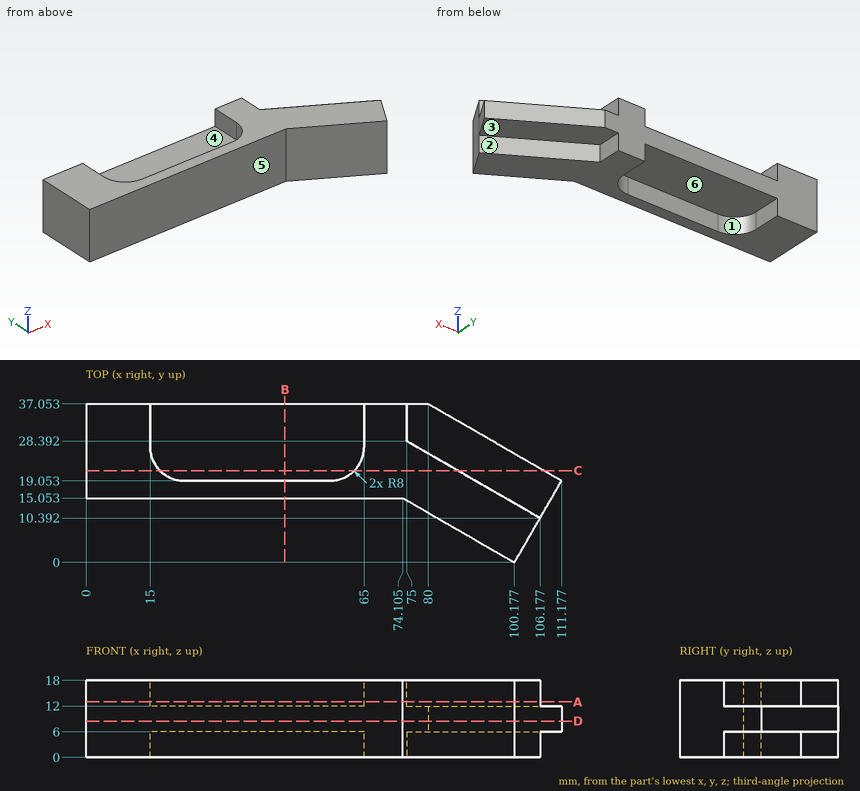
Can you work these out from the drawing? Everything is in mm from the part's minimum corner. A direction names the side the tool comes from. Round coordinates to 2 decimals unless told otherwise and drop trailing zeros. Loops run counter-clockwise (first coordinate to the right, second up) from the corner with the lowest first, then second, coordinate; pieces in that order, holes last. Notation, with made-up numbers: (-40, 68.25) - (-17, 68.25) arc R27 ccw to (-17, 95.25) - close; hole circle Ø10 at (42.5, 14). An arc over 180 degrees is marked (long way). Write item = value, one per line. Start each with the question number.
(1) If I drill on probe 1 along X at (y, z) = (29.5, 14.25); probe 2 along Y at (x, z) = (47.5, 17.5); probe 3 along X at (y, z) = (26, 16) (1 decimal), over which ranges is the centre line in solid material (lowest first)? Write a range as [from, to].
(2) If we section it at D-D (z = 8.5): Please give me the cut outline in (x, y) (1 decimal).
(3) For P1, Ø2, axis at x = 79.5, z = 7.5, coming from the -Y side; P2, Ø14.5, axis at x = 39, y = 24.5, coming from the -Z side; P3, Ø1, axis at x = 43.5, y = 33, coming from the +Z side; P4, Ø3, axis at y = 33.5, z = 2.5, coming from the +X side, each with a flat end and sliding along its axis, tell me the tip position at first contact or that it passes through.
(4) If we section it at B-B (x = 46.5): Please give me the cut outline in (y, z), and give its area (3 significant figures).
(5) If we section it at C-C (y = 21.5): Please give me the cut outline in (x, z), and give its area (3 significant figures).
(6) For the marked faces 4, 5 and 6, which set-ups out of +Z, -Z, +X, -X, +Y, -Y let a thin tool reach every point of the face, with its end or its side?
(7) If we section it at A-A (z = 13): Please give me the cut outline in (x, y) (1 decimal).
(8) If we mould it in two halves opening along X, with no side actions, what happens to the marked faces 1, 2 and 3? For each: released by +X, released by -X, zero draft, split by the parting line, or undercut.
Ans:
q1.probe_1 = [0, 15], [65, 75]
q1.probe_2 = [15.05, 19.05]
q1.probe_3 = [0, 15.1], [64.9, 79.1]
q2.outline = (0, 15.1) - (74.1, 15.1) - (100.2, 0) - (111.2, 19.1) - (80, 37.1) - (0, 37.1) - close
q3.P1 = 11.36
q3.P2 = 0
q3.P3 = 12
q3.P4 = 75
q4.outline = (15.05, 0) - (19.05, 0) - (19.05, 6) - (37.05, 6) - (37.05, 12) - (19.05, 12) - (19.05, 18) - (15.05, 18) - close
q4.area = 180 mm²
q5.outline = (0, 0) - (17.24, 0) - (17.24, 6) - (62.76, 6) - (62.76, 0) - (86.94, 0) - (86.94, 6) - (106.94, 6) - (106.94, 12) - (86.94, 12) - (86.94, 18) - (62.76, 18) - (62.76, 12) - (17.24, 12) - (17.24, 18) - (0, 18) - close
q5.area = 1,140 mm²
q6.face_4 = +Z, +Y
q6.face_5 = +Z, -Z, -X, -Y
q6.face_6 = -Z, +Y
q7.outline = (0, 15.1) - (74.1, 15.1) - (100.2, 0) - (106.2, 10.4) - (75, 28.4) - (75, 37.1) - (65, 37.1) - (65, 27.1) arc R8 cw to (57, 19.1) - (23, 19.1) arc R8 cw to (15, 27.1) - (15, 37.1) - (0, 37.1) - close
q8.face_1 = undercut
q8.face_2 = released by +X
q8.face_3 = zero draft
